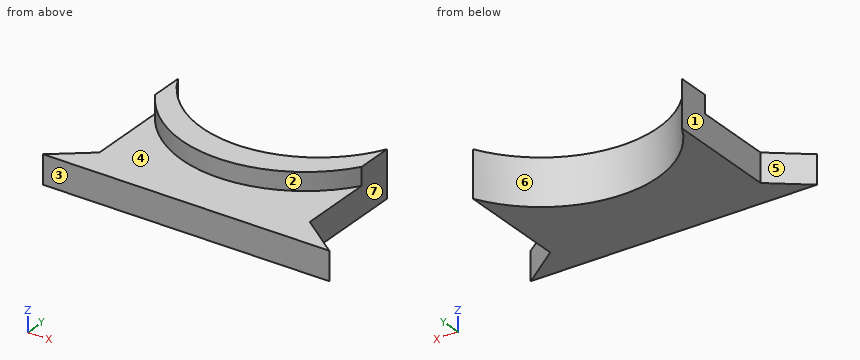
```python
from build123d import *

# Parameters (mm, degrees)
F1_DEPTH      = 8
F3_DEPTH      = 25
F3_DEPTH_BACK = 25
F5_DEPTH      = 5


with BuildPart() as f1:
    # F0 (on Top) → F1 (new body)
    with BuildSketch(Plane.XY):
        Polygon((-45.577269, 28.661994), (-45.577269, -2.913186), (-55.726435, -10.994929), (24.339201, -10.994929), (12.874405, -2.349344), (12.874405, 28.661994), align=None)
    extrude(amount=F1_DEPTH)

    # F2 (on face) → F3 (cut, two sides)
    with BuildSketch(Plane(origin=(0, 0, 0), x_dir=(1, 0, 0), z_dir=(0, 0, -1))) as f3_sk:
        with BuildLine():
            Line((-45.577269, -28.661994), (12.874405, -28.661994))
            ThreePointArc((12.874405, -28.661994), (-16.351432, -10.650162), (-45.577269, -28.661994))
        make_face()
    extrude(amount=-F3_DEPTH, mode=Mode.SUBTRACT)
    extrude(f3_sk.sketch, amount=-F3_DEPTH_BACK, mode=Mode.SUBTRACT)

    # F4 (on face) → F5 (join)
    with BuildSketch(Plane.XY.offset(8)):
        with BuildLine():
            Line((-45.577269, 28.661994), (-45.577269, 19.454254))
            ThreePointArc((-45.577269, 19.454254), (-16.611798, 2.906171), (12.874405, 18.507497))
            Line((12.874405, 18.507497), (12.874405, 28.661994))
            ThreePointArc((12.874405, 28.661994), (-16.351432, 10.650162), (-45.577269, 28.661994))
        make_face()
    extrude(amount=F5_DEPTH)


solid = f1.part
```
Geometry check sheet. Reference: the model listing, model coordinates, mm. Face numbers are marked on the shaded views. A direction names the side the tool comes from. Coordinates: 2 decimals unless noted, no trailing zeros. Loops run counter-clockwise (first coordinate to the right, second up) from the corner with the lowest first, then second, coordinate; pieces in that order, holes last. Notation, with made-up numbers: (40, -35.5) -> (55, -35.5) arc R19 ccw to (55, -6.5) -> close; hole circle Ø3 at (64.5, 1). An arc over 180 degrees is marked (long way). Put each result on its own line as item: value.
1) Gauge pin test, flat ends, axial feed: pin 1 Ø10 at (x, y) = (-3.5, 19) entering from +Z; pin 2 Ø2 at (y, z) = (-6, 5) entering from -X; pin 3 Ø6.5 at (y, z) = (11.5, 5) entering from -X; pin 4 Ø1.5 at (x, y) = (-41.5, 7.5) entering from +Z. Record the tip position at first contact, or that the pin passes through.
Result set:
pin 1: passes through
pin 2: stops at x = -50.71
pin 3: stops at x = -45.58
pin 4: stops at z = 8
2) Cross-section at B-B on z = 7. Record the boundary of the cut face in (x, y).
Result set:
outline: (-55.73, -10.99) -> (24.34, -10.99) -> (12.87, -2.35) -> (12.87, 28.66) arc R32.72 cw to (-45.58, 28.66) -> (-45.58, -2.91) -> close
3) Thickness scan on line 1 (Z direction, x = -1, y = -7.5); line 2 (X direction, y = 14, z = 9.25); line 3 (X direction, y = 0, z = 3.75). Record the ranges inside material, lowest first.
Result set:
line 1: z = 0 to 8
line 2: x = -41.45 to -30.77, -1.93 to 9.35
line 3: x = -45.58 to 12.87
4) Tool access check on the marked faces 1, 2 and 3. Record the directions out of +Z, -Z, +X, -X, +Y, -Y that give a thin tool (end or side, any length) a straight path to the whole face; none if there is none.
Result set:
face 1: +Z, -Z, -X, +Y
face 2: +Z, -Y
face 3: +Z, -Z, +X, -X, -Y
5) Cross-section at A-A on y = 25. Record the boundary of the cut face in (x, z), plus the area to 3 significant figures.
Result set:
outline: (-45.58, 0) -> (-43.43, 0) -> (-43.43, 13) -> (-45.58, 13) -> close; (10.72, 0) -> (12.87, 0) -> (12.87, 13) -> (10.72, 13) -> close
area: 55.9 mm^2
6) Cross-section at D-D on y = 2. Record the boundary of the cut face in (x, z).
Result set:
outline: (-45.58, 0) -> (12.87, 0) -> (12.87, 8) -> (-45.58, 8) -> close
7) Release check for a two-part mould opening along X. For the marked faces 4, 5, 6 and 7 record: released by +X, released by -X, zero draft, split by the parting line, or undercut.
Result set:
face 4: zero draft
face 5: released by -X
face 6: undercut
face 7: released by +X
8) Cross-section at C-C on x = -21.5. Record the boundary of the cut face in (y, z).
Result set:
outline: (-10.99, 0) -> (11.06, 0) -> (11.06, 13) -> (3.33, 13) -> (3.33, 8) -> (-10.99, 8) -> close
